Drawing for the job (mm, zero at the part's lowest x, y, z). Give positions to 0.01 mm unless a question says otherwise; leave off trailing zeros. Order: outer loops, then holes, each group sorted by start corner. A loop starts at its lowest first (then second) coordinate and runs counter-clockwise, first axis right, second up. Notation, with made-up numbers: (17.25, 82.25) -> (43.25, 82.25) arc R27 ccw to (43.25, 114.25) -> close; hole circle Ø4 at (-17, 33.25). An arc over 180 degrees is marked (long way). Use one line per item in the form item = value. Start each with the question number.
1) Cut at A-A, the plane x = 124.26. Give the cut face in (y, z) (3 decimals), and give its area (3 significant figures).
2) Probe line 1 (Y direction, x = 124.26, z = 10.25) (3 decimals); line 2 (Y direction, x = 109, z = 101) (3 decimals); line 3 (Z direction, x = 11.5, y = 8.25). List the from-to ranges inside material, lowest first.
3) Mould opens along X. For the marked faces 1, 2 and 3 say: pulls with the +X half, pulls with the -X half, needs draft (parallel to the pull), parting line crosses it, or undercut.
4) Drop flat-ended pins along their axis: P1, Ø6, axis at x = 15.24, y = 9.325, coming from the +Z side; P2, Ø1.9, axis at y = 5.5, z = 4, coming from the +X side; P3, Ø12, axis at x = 47.5, z = 50.5, coming from the +Y side (3 decimals); P4, Ø5, axis at x = 25.5, y = 11, coming from the -Z side. Give the stop position or say it passes through.
5) Cut at C-C, the plane x = 50. Give the cut face in (y, z) (3 decimals).
6) Cut at B-B, the plane z = 54.5. Give the cut face in (x, y) (3 decimals), and give its area (3 significant figures).
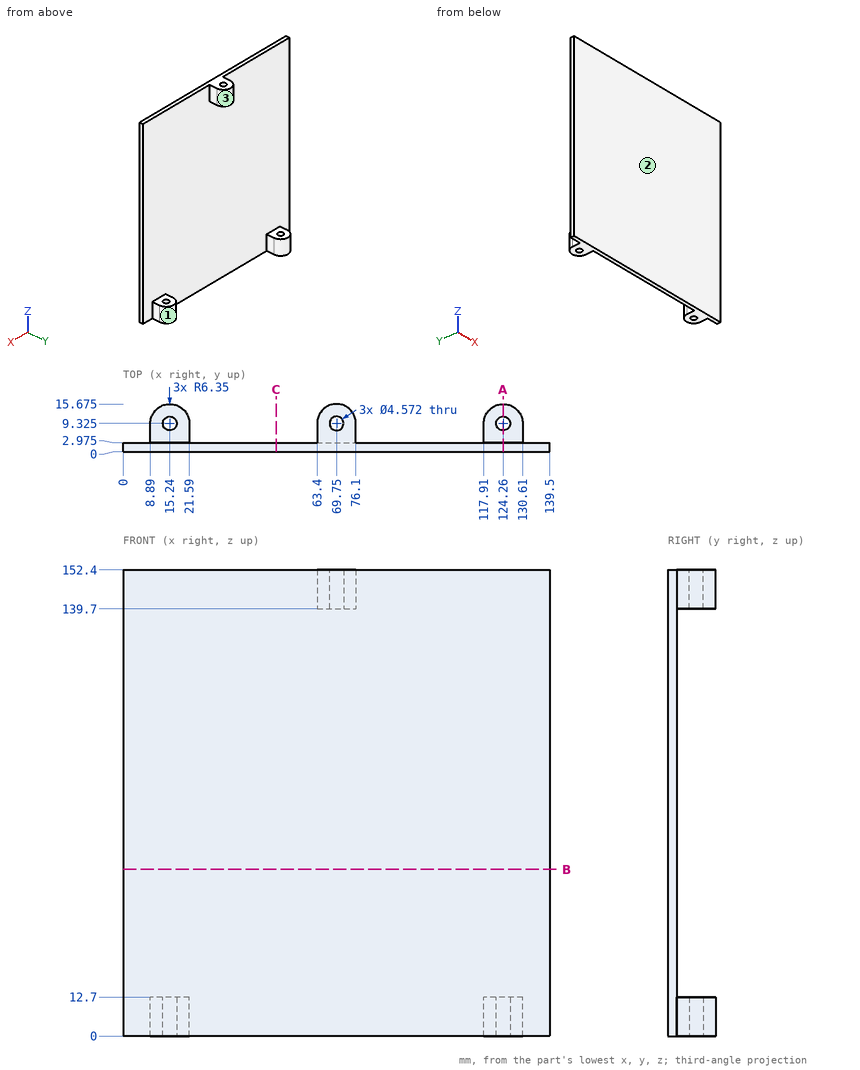
Result:
q1.outline = (0, 0) -> (7.039, 0) -> (7.039, 12.7) -> (2.975, 12.7) -> (2.975, 152.4) -> (0, 152.4) -> close; (11.611, 0) -> (15.675, 0) -> (15.675, 12.7) -> (11.611, 12.7) -> close
q1.area = 557 mm²
q2.line_1 = 0 to 7.039, 11.611 to 15.675
q2.line_2 = 0 to 2.975
q2.line_3 = 0 to 12.7
q3.face_1 = undercut
q3.face_2 = needs draft
q3.face_3 = parting line crosses it
q4.P1 = 12.7
q4.P2 = 130.61
q4.P3 = 2.975
q4.P4 = through
q5.outline = (0, 0) -> (2.975, 0) -> (2.975, 152.4) -> (0, 152.4) -> close
q6.outline = (0, 0) -> (139.5, 0) -> (139.5, 2.975) -> (0, 2.975) -> close
q6.area = 415 mm²
